from build123d import *

# Parameters (mm, degrees)
BOSS_EXTRUDE1_DEPTH = 4
CUT_EXTRUDE1_DEPTH  = 10


with BuildPart() as part:
    # Sketch1 → Boss-Extrude1 (new body)
    with BuildSketch(Plane.XY):
        with BuildLine():
            ThreePointArc((0.432215106, 6.121703644), (-0.006111672, 5.480502071), (0, 4.703821656))
            ThreePointArc((0, 4.703821656), (-0.335566795, 4.691836858), (-0.669423618, 4.655943534))
            ThreePointArc((-0.669423618, 4.655943534), (-0.773907302, 5.425588244), (-1.299025043, 5.997882904))
            ThreePointArc((-1.299025043, 5.997882904), (0.437804478, -6.121306449), (0.432215106, 6.121703644))
        make_face()
    extrude(amount=BOSS_EXTRUDE1_DEPTH)

    # Sketch2 → Cut-Extrude1 (cut)
    with BuildSketch(Plane.XY.offset(4)):
        with BuildLine():
            ThreePointArc((-3.554911214, 3.080348102), (-4.145889401, 3.584346716), (-4.343434222, 4.335509723))
            ThreePointArc((-4.343434222, 4.335509723), (-4.912875705, 3.677732686), (-5.383577945, 2.946040378))
            ThreePointArc((-5.383577945, 2.946040378), (-4.60718751, 2.968124585), (-3.957106586, 2.543077985))
            ThreePointArc((-3.957106586, 2.543077985), (-3.765603226, 2.818895266), (-3.554911214, 3.080348102))
        make_face()
        with BuildLine():
            ThreePointArc((-2.543077985, 3.957106586), (-2.968124585, 4.60718751), (-2.946040378, 5.383577945))
            ThreePointArc((-2.946040378, 5.383577945), (-3.677732686, 4.912875705), (-4.335509723, 4.343434222))
            ThreePointArc((-4.335509723, 4.343434222), (-3.584346716, 4.145889401), (-3.080348102, 3.554911214))
            ThreePointArc((-3.080348102, 3.554911214), (-2.818895266, 3.765603226), (-2.543077985, 3.957106586))
        make_face()
        with BuildLine():
            ThreePointArc((-1.325219702, 4.513283828), (-1.549899967, 5.256781372), (-1.309975863, 5.995500699))
            ThreePointArc((-1.309975863, 5.995500699), (-2.144641637, 5.750006752), (-2.936204288, 5.388948857))
            ThreePointArc((-2.936204288, 5.388948857), (-2.271123467, 4.987778915), (-1.954038134, 4.278746679))
            ThreePointArc((-1.954038134, 4.278746679), (-1.643817176, 4.407244407), (-1.325219702, 4.513283828))
        make_face()
        with BuildLine():
            ThreePointArc((2.139390577, 5.751962566), (1.304500997, 5.996694302), (0.443393485, 6.12090415))
            ThreePointArc((0.443393485, 6.12090415), (0.78600623, 5.423848681), (0.669423618, 4.655943534))
            ThreePointArc((0.669423618, 4.655943534), (0.999869212, 4.596324589), (1.325219702, 4.513283828))
            ThreePointArc((1.325219702, 4.513283828), (1.538171755, 5.260225086), (2.139390577, 5.751962566))
        make_face()
        with BuildLine():
            ThreePointArc((3.673245347, 4.916231689), (2.941123559, 5.386265646), (2.14989091, 5.748046144))
            ThreePointArc((2.14989091, 5.748046144), (2.282242211, 4.982701155), (1.954038134, 4.278746679))
            ThreePointArc((1.954038134, 4.278746679), (2.254301762, 4.128445438), (2.543077985, 3.957106586))
            ThreePointArc((2.543077985, 3.957106586), (2.957841655, 4.613795948), (3.673245347, 4.916231689))
        make_face()
        with BuildLine():
            ThreePointArc((4.909515624, 3.682216959), (4.339473781, 4.339473781), (3.682216959, 4.909515624))
            ThreePointArc((3.682216959, 4.909515624), (3.593584502, 4.137884814), (3.080348102, 3.554911214))
            ThreePointArc((3.080348102, 3.554911214), (3.32610419, 3.32610419), (3.554911214, 3.080348102))
            ThreePointArc((3.554911214, 3.080348102), (4.137884814, 3.593584502), (4.909515624, 3.682216959))
        make_face()
        with BuildLine():
            ThreePointArc((5.748046144, 2.14989091), (5.386265646, 2.941123559), (4.916231689, 3.673245347))
            ThreePointArc((4.916231689, 3.673245347), (4.613795948, 2.957841655), (3.957106586, 2.543077985))
            ThreePointArc((3.957106586, 2.543077985), (4.128445438, 2.254301762), (4.278746679, 1.954038134))
            ThreePointArc((4.278746679, 1.954038134), (4.982701155, 2.282242211), (5.748046144, 2.14989091))
        make_face()
        with BuildLine():
            ThreePointArc((6.12090415, 0.443393485), (5.996694302, 1.304500997), (5.751962566, 2.139390577))
            ThreePointArc((5.751962566, 2.139390577), (5.260225086, 1.538171755), (4.513283828, 1.325219702))
            ThreePointArc((4.513283828, 1.325219702), (4.596324589, 0.999869212), (4.655943534, 0.669423618))
            ThreePointArc((4.655943534, 0.669423618), (5.423848681, 0.78600623), (6.12090415, 0.443393485))
        make_face()
        with BuildLine():
            ThreePointArc((5.997882904, -1.299025043), (6.121306449, -0.437804478), (6.121703644, 0.432215106))
            ThreePointArc((6.121703644, 0.432215106), (5.480502071, -0.006111672), (4.703821656, 0))
            ThreePointArc((4.703821656, 0), (4.691836858, -0.335566795), (4.655943534, -0.669423618))
            ThreePointArc((4.655943534, -0.669423618), (5.425588244, -0.773907302), (5.997882904, -1.299025043))
        make_face()
        with BuildLine():
            ThreePointArc((5.388948857, -2.936204288), (5.750006752, -2.144641637), (5.995500699, -1.309975863))
            ThreePointArc((5.995500699, -1.309975863), (5.256781372, -1.549899967), (4.513283828, -1.325219702))
            ThreePointArc((4.513283828, -1.325219702), (4.407244407, -1.643817176), (4.278746679, -1.954038134))
            ThreePointArc((4.278746679, -1.954038134), (4.987778915, -2.271123467), (5.388948857, -2.936204288))
        make_face()
        with BuildLine():
            ThreePointArc((4.343434222, -4.335509723), (4.912875705, -3.677732686), (5.383577945, -2.946040378))
            ThreePointArc((5.383577945, -2.946040378), (4.60718751, -2.968124585), (3.957106586, -2.543077985))
            ThreePointArc((3.957106586, -2.543077985), (3.765603226, -2.818895266), (3.554911214, -3.080348102))
            ThreePointArc((3.554911214, -3.080348102), (4.145889401, -3.584346716), (4.343434222, -4.335509723))
        make_face()
        with BuildLine():
            ThreePointArc((2.946040378, -5.383577945), (3.677732686, -4.912875705), (4.335509723, -4.343434222))
            ThreePointArc((4.335509723, -4.343434222), (3.584346716, -4.145889401), (3.080348102, -3.554911214))
            ThreePointArc((3.080348102, -3.554911214), (2.818895266, -3.765603226), (2.543077985, -3.957106586))
            ThreePointArc((2.543077985, -3.957106586), (2.968124585, -4.60718751), (2.946040378, -5.383577945))
        make_face()
        with BuildLine():
            ThreePointArc((1.309975863, -5.995500699), (2.144641637, -5.750006752), (2.936204288, -5.388948857))
            ThreePointArc((2.936204288, -5.388948857), (2.271123467, -4.987778915), (1.954038134, -4.278746679))
            ThreePointArc((1.954038134, -4.278746679), (1.643817176, -4.407244407), (1.325219702, -4.513283828))
            ThreePointArc((1.325219702, -4.513283828), (1.549899967, -5.256781372), (1.309975863, -5.995500699))
        make_face()
        with BuildLine():
            ThreePointArc((0, -4.703821656), (0.006111672, -5.480502071), (-0.432215106, -6.121703644))
            ThreePointArc((-0.432215106, -6.121703644), (0.437804478, -6.121306449), (1.299025043, -5.997882904))
            ThreePointArc((1.299025043, -5.997882904), (0.773907302, -5.425588244), (0.669423618, -4.655943534))
            ThreePointArc((0.669423618, -4.655943534), (0.335566795, -4.691836858), (0, -4.703821656))
        make_face()
        with BuildLine():
            ThreePointArc((-1.325219702, -4.513283828), (-1.538171755, -5.260225086), (-2.139390577, -5.751962566))
            ThreePointArc((-2.139390577, -5.751962566), (-1.304500997, -5.996694302), (-0.443393485, -6.12090415))
            ThreePointArc((-0.443393485, -6.12090415), (-0.78600623, -5.423848681), (-0.669423618, -4.655943534))
            ThreePointArc((-0.669423618, -4.655943534), (-0.999869212, -4.596324589), (-1.325219702, -4.513283828))
        make_face()
        with BuildLine():
            ThreePointArc((-2.543077985, -3.957106586), (-2.957841655, -4.613795948), (-3.673245347, -4.916231689))
            ThreePointArc((-3.673245347, -4.916231689), (-2.941123559, -5.386265646), (-2.14989091, -5.748046144))
            ThreePointArc((-2.14989091, -5.748046144), (-2.282242211, -4.982701155), (-1.954038134, -4.278746679))
            ThreePointArc((-1.954038134, -4.278746679), (-2.254301762, -4.128445438), (-2.543077985, -3.957106586))
        make_face()
        with BuildLine():
            ThreePointArc((-3.554911214, -3.080348102), (-4.137884814, -3.593584502), (-4.909515624, -3.682216959))
            ThreePointArc((-4.909515624, -3.682216959), (-4.339473781, -4.339473781), (-3.682216959, -4.909515624))
            ThreePointArc((-3.682216959, -4.909515624), (-3.593584502, -4.137884814), (-3.080348102, -3.554911214))
            ThreePointArc((-3.080348102, -3.554911214), (-3.32610419, -3.32610419), (-3.554911214, -3.080348102))
        make_face()
        with BuildLine():
            ThreePointArc((-4.278746679, -1.954038134), (-4.982701155, -2.282242211), (-5.748046144, -2.14989091))
            ThreePointArc((-5.748046144, -2.14989091), (-5.386265646, -2.941123559), (-4.916231689, -3.673245347))
            ThreePointArc((-4.916231689, -3.673245347), (-4.613795948, -2.957841655), (-3.957106586, -2.543077985))
            ThreePointArc((-3.957106586, -2.543077985), (-4.128445438, -2.254301762), (-4.278746679, -1.954038134))
        make_face()
        with BuildLine():
            ThreePointArc((-4.655943534, -0.669423618), (-5.423848681, -0.78600623), (-6.12090415, -0.443393485))
            ThreePointArc((-6.12090415, -0.443393485), (-5.996694302, -1.304500997), (-5.751962566, -2.139390577))
            ThreePointArc((-5.751962566, -2.139390577), (-5.260225086, -1.538171755), (-4.513283828, -1.325219702))
            ThreePointArc((-4.513283828, -1.325219702), (-4.596324589, -0.999869212), (-4.655943534, -0.669423618))
        make_face()
        with BuildLine():
            ThreePointArc((-4.655943534, 0.669423618), (-5.425588244, 0.773907302), (-5.997882904, 1.299025043))
            ThreePointArc((-5.997882904, 1.299025043), (-6.121306449, 0.437804478), (-6.121703644, -0.432215106))
            ThreePointArc((-6.121703644, -0.432215106), (-5.480502071, 0.006111672), (-4.703821656, 0))
            ThreePointArc((-4.703821656, 0), (-4.691836858, 0.335566795), (-4.655943534, 0.669423618))
        make_face()
        with BuildLine():
            ThreePointArc((-4.278746679, 1.954038134), (-4.987778915, 2.271123467), (-5.388948857, 2.936204288))
            ThreePointArc((-5.388948857, 2.936204288), (-5.750006752, 2.144641637), (-5.995500699, 1.309975863))
            ThreePointArc((-5.995500699, 1.309975863), (-5.256781372, 1.549899967), (-4.513283828, 1.325219702))
            ThreePointArc((-4.513283828, 1.325219702), (-4.407244407, 1.643817176), (-4.278746679, 1.954038134))
        make_face()
    extrude(amount=-CUT_EXTRUDE1_DEPTH, mode=Mode.SUBTRACT)


solid = part.part
The model under review builds one solid part; all positions refer to its coordinate system, in mm. Coordinates: 2 decimals unless noted, no trailing zeros. Loops run counter-clockwise (first coordinate to the right, second up) from the corner with the lowest first, then second, coordinate; pieces in that order, holes last. Notation, with made-up numbers: (5, -13) -> (16, -13) arc R15 ccw to (16, -7) -> close; hole circle Ø4 at (8.25, -38.5). An arc over 180 degrees is marked (long way). Use a Markdown table: item, result. Add a question column.
1. To check wall thickness, follow line 1 (X direction, y = -5, z = 3.2); line 2 (Y direction, x = 4.75, z = 0.35); line 3 (Y direction, x = -5.25, z = 3.3). State the ranges of each line that lie inside material, in increasing order.
2. Add section B-B on x = -1.75. Write out the cut boundary in (y, z).
3. Add section A-A on x = 3.25. Write out the cut boundary in (y, z), plus the area to 3 significant figures.
4. Draft analysis for pull direction Y (two halves, no side actions). For faces 1 (the face through (5.42, -0.77, 2.03)), 2 (the face through (4.14, -3.575, 2.028)), state which applies: pulls with the +Y half, pulls with the -Y half, needs draft (parallel to the pull), parting line crosses it, or undercut.
5. Clearance check with a flat-ended pin moving along its axis: pin 1 Ø2 at (y, z) = (-1.5, 2) entering from +X. State where the tip first meets the part, or that it passes through.
Returned:
| question | item | result |
|---|---|---|
| 1 | line 1 | x = -2.28 to -1.41, -0.78 to 0.06, 0.66 to 1.53, 2.28 to 3.02 |
| 1 | line 2 | y = -3 to -2.1, -1.45 to -0.66, -0.01 to 0.71, 1.34 to 2.23, 3.15 to 3.7 |
| 1 | line 3 | y = -2.29 to -1.53, -0.8 to 0.05, 0.71 to 1.55, 2.59 to 2.98 |
| 2 | outline | (-5.51, 0) -> (4.37, 0) -> (4.37, 4) -> (-5.51, 4) -> close |
| 3 | outline | (-3.84, 0) -> (3.4, 0) -> (3.4, 4) -> (-3.84, 4) -> close; (3.68, 0) -> (4.8, 0) -> (4.8, 4) -> (3.68, 4) -> close |
| 3 | area | 33.5 mm² |
| 4 | face 1 | undercut |
| 4 | face 2 | undercut |
| 5 | pin 1 | stops at x = 6 |
